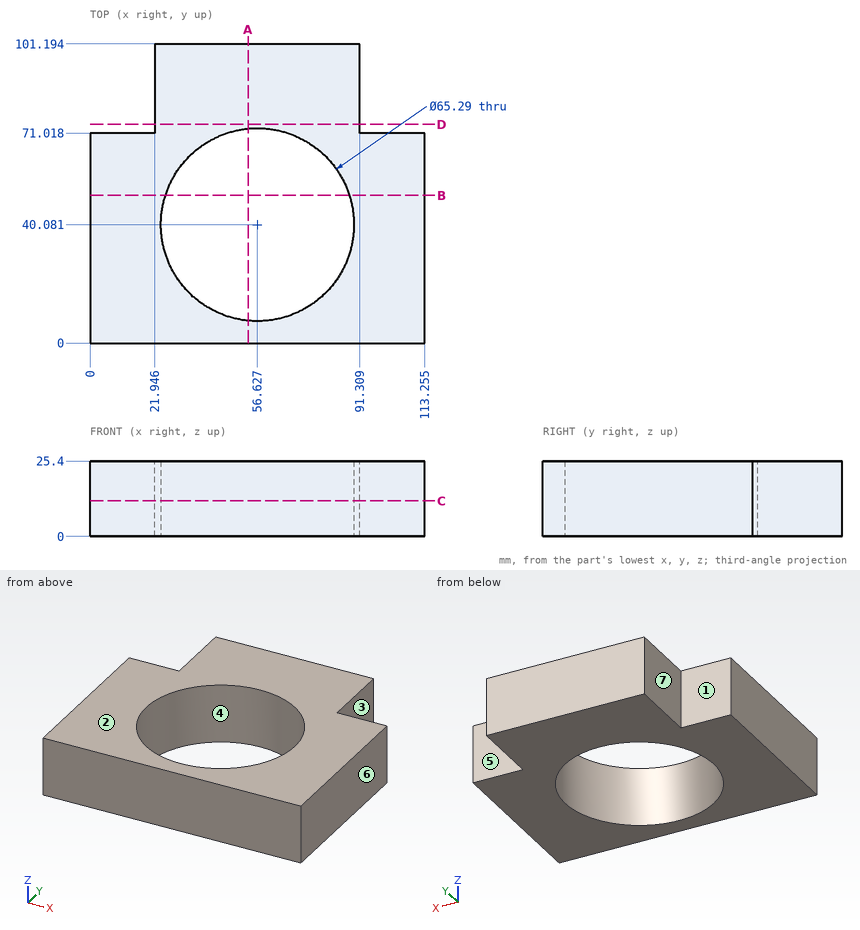
Verification items for this drawing (mm, ordinates from the low corner). A direction names the side the tool comes from. Coordinates: 2 decimals unless noted, no trailing zeros. Write each loop counter-clockwise with the first axis right and the second up, starting at its lowest first coordinate (ties: lowest second). Pieces come first, ordered by that corner, then holes. Notation, with made-up numbers: M -33,32.5 L -3,32.5 A9 cw -3,42.5 Z; hole C 74.25,5 d11. An arc over 180 degrees is marked long. Use one line per item in the form item = value. Start each with the question number.
1) Release check for a two-part mould opening along X. For the marked faces 4, 5, 6 and 7 record: pulls with the +X half, pulls with the -X half, needs draft (parallel to the pull), parting line crosses it, or undercut.
2) Section check A-A on x = 53.5. Enter the section's corners in (y, z).
3) Section check B-B on y = 50. Enter the section's corners in (x, z) (1 decimal), and give its area (3 significant figures).
4) Go/stop test with flat-tipped pins: pin 1 Ø7.5 at (y, z) = (90.5, 19) entering from +X; pin 2 Ø11 at (x, z) = (10, 11.5) entering from +Y; pin 3 Ø6 at (y, z) = (90.5, 13.5) entering from -X. Record where each tip stops, or that it passes through.
5) Section check D-D on y = 74. Enter the section's corners in (x, z) (1 decimal), and give its area (3 significant figures).
6) Set-up check for the marked faces 1, 2 and 3: record each of +Z, -Z, +X, -X, +Y, -Y from which the full face is reachable in a straight line by a thin tool's end or side.
7) Section check C-C on z = 12. Enter the section's corners in (x, y) (1 decimal).
8) Thickness scan on probe 1 along X at (y, z) = (94, 13) (1 decimal); probe 2 along Y at (x, z) = (81.5, 10.5) (1 decimal); probe 3 along X at (y, z) = (12, 11) (1 decimal). Record the ranges inside material, lowest first. Write a range as from..to.
Responses:
q1.face_4 = undercut
q1.face_5 = needs draft
q1.face_6 = pulls with the +X half
q1.face_7 = pulls with the -X half
q2.outline = M 0,0 L 7.59,0 L 7.59,25.4 L 0,25.4 Z; M 72.58,0 L 101.19,0 L 101.19,25.4 L 72.58,25.4 Z
q3.outline = M 0,0 L 25.5,0 L 25.5,25.4 L 0,25.4 Z; M 87.7,0 L 113.3,0 L 113.3,25.4 L 87.7,25.4 Z
q3.area = 1,300 mm2
q4.pin_1 = 91.31
q4.pin_2 = 71.02
q4.pin_3 = 21.95
q5.outline = M 21.9,0 L 91.3,0 L 91.3,25.4 L 21.9,25.4 Z
q5.area = 1,760 mm2
q6.face_1 = +Z, -Z, -X, +Y
q6.face_2 = +Z, +X, -X, +Y, -Y
q6.face_3 = +Z, -Z, +X, +Y
q7.outline = M 0,0 L 113.3,0 L 113.3,71 L 91.3,71 L 91.3,101.2 L 21.9,101.2 L 21.9,71 L 0,71 Z; hole C 56.6,40.1 d65.3
q8.probe_1 = 21.9..91.3
q8.probe_2 = 0..18.9, 61.2..101.2
q8.probe_3 = 0..40, 73.3..113.3
